For this review, take the finished solid that the model builds, in its own axes (mm). Give positions to 0.01 mm unless a question says otherwise; leave off trailing zeros. Loops run counter-clockwise (first coordinate to the right, second up) from the corner with the lowest first, then second, coordinate; pieces in that order, holes last.
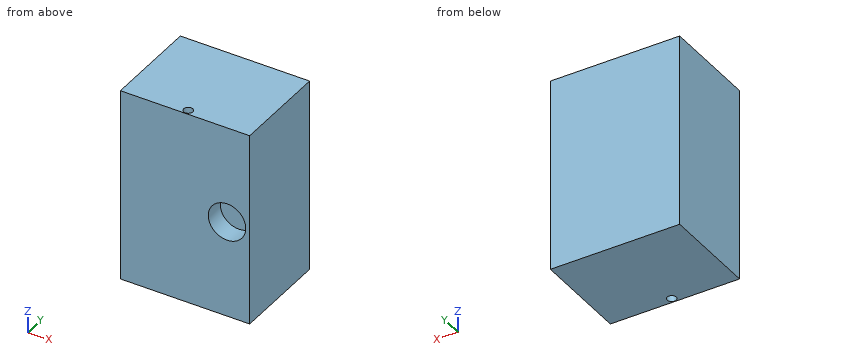
Autodesk Inventor part; units mm, degrees
ref_plane "YZ Plane" through (0, 0, 0) normal (1, 0, 0) x (0, 1, 0)
ref_plane "XZ Plane" through (0, 0, 0) normal (0, 1, 0) x (-1, 0, 0)
ref_plane "XY Plane" through (0, 0, 0) normal (0, 0, 1) x (1, 0, 0)
sketch "Sketch1" plane through (0, 0, 0) normal (0, 1, 0) x (-1, 0, 0)
  line L0 (0, 0) -> (100, 0)
  line L1 (100, 0) -> (100, -150)
  line L2 (100, -150) -> (0, -150)
  line L3 (0, -150) -> (0, 0)
  dimension "d0" = 100
  dimension "d1" = 150
extrude "Extrusion1" add sketch "Sketch1" along normal blind 75
sketch "Sketch2" plane through (0, 0, -150) normal (0, 0, -1) x (-1, 0, 0)
  line L0 (0, 0) -> (100, 0)
  circle A0 centre (50, 4) radius 3.5
hole "Hole1" at (-50, 4, -150) direction (0, 0, 1) diameter 7 depth 8
sketch "Sketch3" plane through (-100, 0, 0) normal (0, 0, 1) x (1, 0, 0)
  circle A0 centre (50, 4) radius 3.5
  circle A1 centre (50, 4) radius 3.5
  point P0 (100, 0)
hole "Hole2" at (-50, 4, 0) direction (0, 0, -1) diameter 7 depth 8
sketch "Sketch4" plane through (0, 0, 0) normal (0, -1, 0) x (1, 0, 0)
  point P0 (0, 0)
sketch "Sketch5" plane through (0, 0, 0) normal (0, -1, 0) x (1, 0, 0)
  line L0 (0, 0) -> (0, -150)
  line L1 (0, -75) -> (-100, -75)
  line L2 (-100, -150) -> (-100, 0)
sketch "Sketch6" plane through (0, 0, 0) normal (0, -1, 0) x (1, 0, 0)
  circle A0 centre (-17.5284, -75) radius 15
  point P0 (0, 0)
  dimension "d20" = 30
hole "Hole3" at (-17.5284, 0, -75) direction (0, 1, 0) diameter 29 depth 15
properties part number "Box 1"
Item 1: Take a section at A-A on y = 4. Give the boundary of the cut face in (x, z).
Answer:
outline: (-100, -150) - (-53.5, -150) - (-53.5, -142) - (-46.5, -142) - (-46.5, -150) - (0, -150) - (0, 0) - (-46.5, 0) - (-46.5, -8) - (-53.5, -8) - (-53.5, 0) - (-100, 0) - close; hole circle Ø29 at (-17.53, -75)
Item 2: Take a section at C-C on x = -14.5. Give the boundary of the cut face in (y, z).
Answer:
outline: (0, -150) - (75, -150) - (75, 0) - (0, 0) - (0, -60.82) - (15, -60.82) - (15, -89.18) - (0, -89.18) - close
Item 3: Take a section at B-B on z = -75. Give the boundary of the cut face in (x, y), and give its area (4 significant figures).
Answer:
outline: (-100, 0) - (-32.03, 0) - (-32.03, 15) - (-3.03, 15) - (-3.03, 0) - (0, 0) - (0, 75) - (-100, 75) - close
area: 7,065 mm2
Item 4: Clearance check with flat-ended pins moving along their axes: pin 1 Ø6.5 at (x, y) = (-50, 4) entering from +Z; pin 2 Ø17.5 at (x, z) = (-17.53, -75) entering from -Y; pin 3 Ø3.5 at (x, y) = (-49.5, 2.5) entering from -Z. State where each tip first meets the part, or that it passes through.
Answer:
pin 1: stops at z = -8
pin 2: stops at y = 15
pin 3: stops at z = -142
Item 5: For L1, parallel to X at y = 7.25, z = -75; L2, parallel to X at y = 4, z = -1.5; L3, parallel to Z at x = -17, y = 11, list the stretches that pass through material, from the lowest coordinate up.
Answer:
L1: x = -100 to -32.03, -3.03 to 0
L2: x = -100 to -53.5, -46.5 to 0
L3: z = -150 to -89.49, -60.51 to 0
